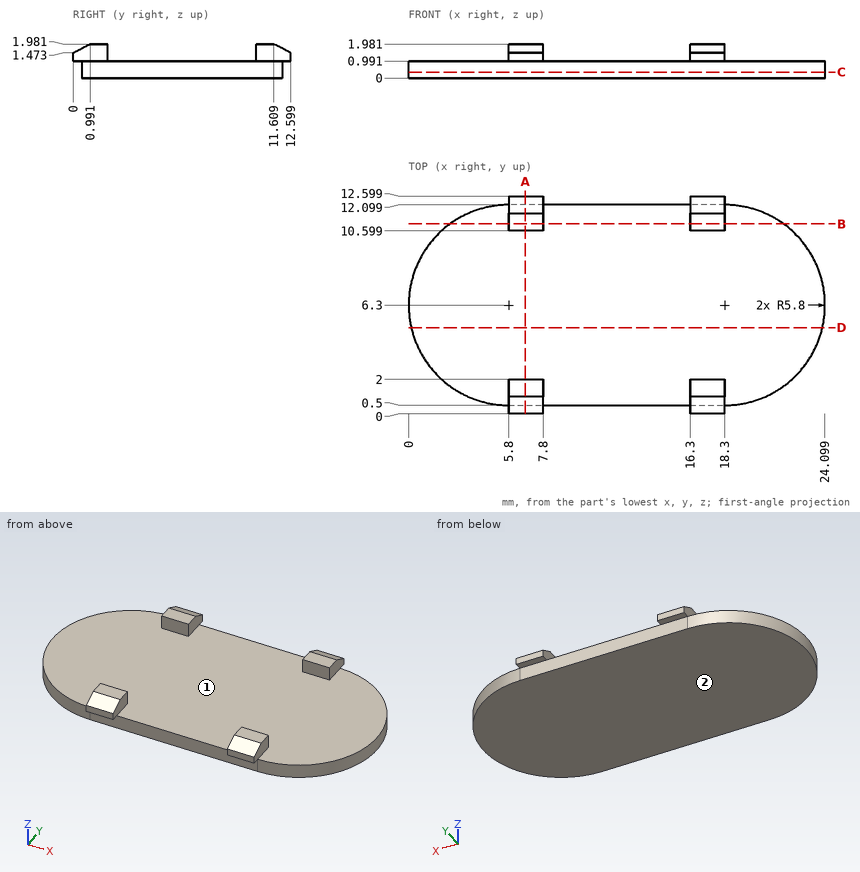
Check sheet for the drawn part. Datum: minimum x, y, z corner. Units: mm. Round coordinates to 2 decimals unless told otherwise and drop trailing zeros. Order: outer loops, then holes, each group sorted by start corner. A loop starts at its lowest first (then second) coordinate and runs counter-clockwise, first axis right, second up. Notation, with made-up numbers: M 9.5,28.25 L 65.5,28.25 A20 ccw 65.5,51.25 Z; hole C 11.5,66.25 d10. An arc over 180 degrees is marked long. Write each question's results on one line, items separated by ' | '. Start each with the question number.
1. Cross-section at C-C on z = 0.35. Record the boundary of the cut face in (x, y), plus the area to 3 significant figures.
2. Draft check along Y on the marked faces 1 and 2. Enter one of: pulls with the +Y half, pulls with the -Y half, needs draft (parallel to the pull), parting line crosses it, or undercut.
3. Cross-section at D-D on y = 5. Record the boundary of the cut face in (x, z).
4. Material ranges on L1, parallel to X at y = 11.5, z = 1.1; L2, parallel to Z at x = 5.25, y = 10.5; L3, parallel to Y at x = 17, z = 1.3, recorded low to high. Write a range as from..to.
5. Cross-section at A-A on x = 6.75. Record the boundary of the cut face in (y, z).
6. Cross-section at B-B on y = 11. Record the boundary of the cut face in (x, z).
7. Go/stop test with flat-tipped pins: P1, Ø0.8, axis at y = 12, z = 1.5, coming from the +X side; P2, Ø0.5, axis at y = 12, z = 1.5, coming from the -X side; P3, Ø4, axis at x = 5, y = 6, coming from the +Z side. Record where each tip stops, or that it passes through.
Resolved:
1) outline: M 5.8,0.5 L 18.3,0.5 A5.8 ccw 18.3,12.1 L 5.8,12.1 A5.8 ccw Z | area: 251 mm2
2) face 1: undercut | face 2: needs draft
3) outline: M 0.15,0 L 23.95,0 L 23.95,0.99 L 0.15,0.99 Z
4) L1: 5.8..7.8, 16.3..18.3 | L2: 0..0.99 | L3: 0..2, 10.6..12.6
5) outline: M 0,0.99 L 0.5,0.99 L 0.5,0 L 12.1,0 L 12.1,0.99 L 12.6,0.99 L 12.6,1.47 L 11.61,1.98 L 10.6,1.98 L 10.6,0.99 L 2,0.99 L 2,1.98 L 0.99,1.98 L 0,1.47 Z
6) outline: M 2.4,0 L 21.7,0 L 21.7,0.99 L 18.3,0.99 L 18.3,1.98 L 16.3,1.98 L 16.3,0.99 L 7.8,0.99 L 7.8,1.98 L 5.8,1.98 L 5.8,0.99 L 2.4,0.99 Z
7) P1: x = 18.3 | P2: x = 5.8 | P3: z = 0.99
